The listing builds one solid part. Answer for the finished solid, in the listing's coordinates (mm). Coordinates: 2 decimals unless noted, no trailing zeros. Order: outer loops, then holes, each group sorted by start corner. A loop starts at its lowest first (then second) coordinate and runs counter-clockwise, first axis right, second up. Notation, with made-up numbers: (80, 31) - (92, 31) arc R13 cw to (92, 39) - close; hole circle Ø7 at (51.5, -33.75). An arc over 180 degrees is marked (long way). Use a Markdown table: item, result. Add a question column.
Item 1: Find the intervals of material crossed by line 1 along Y through (x, z) = (1.75, 8); line 2 along Y through (x, z) = (6.5, -23), in increasing order.
Item 2: Flat-ended cylindrical pins translate along their axes: P1, Ø3.5, axis at y = 23, z = 0, coming from the -X side; P2, Ø3, axis at x = 5.5, z = 13, coming from the +Y side; P3, Ø1, axis at x = 3, y = 30, coming from the -Z side. Find the tip coordinate at first contact, or state that the pin passes through.
Item 3: The part is cut by section A-A, the plane z = 0. Give the vertices of the cut face in (x, y).
Item 4: The part is cut by section B-B, the plane x = 6. State how many separate pieces and enclosed holes the cut face has, then the cut area to 3 significant figures.
from build123d import *

# Parameters (mm, degrees)
SPROCKET_R                   = 45.25
ESTRUSIONE_ESTRUSIONE2_DEPTH = 8
SCHIZZO1_R                   = 5
SCHIZZO1_R_2                 = 1.5
TAGLIO_ESTRUSIONE2_DEPTH     = 9
RACCORDO1_R                  = 0.5


with BuildPart() as part:
    # Sprocket → Estrusione-Estrusione2 (new body)
    with BuildSketch(Plane(origin=(0, 0, 0), x_dir=(0, 0, -1), z_dir=(1, 0, 0))):
        Circle(SPROCKET_R)
    extrude(amount=ESTRUSIONE_ESTRUSIONE2_DEPTH)

    # Schizzo1 → Taglio-Estrusione2 (cut, through all)
    with BuildSketch(Plane(origin=(0, 0, 0), x_dir=(0, 0, -1), z_dir=(1, 0, 0))):
        Circle(SCHIZZO1_R)
        with Locations((0, 23)):
            Circle(SCHIZZO1_R_2)
        with Locations((8, 0)):
            Circle(SCHIZZO1_R_2)
        with Locations((0, 8)):
            Circle(SCHIZZO1_R_2)
        with Locations((23, 0)):
            Circle(SCHIZZO1_R_2)
        with Locations((0, -8)):
            Circle(SCHIZZO1_R_2)
        with Locations((0, -23)):
            Circle(SCHIZZO1_R_2)
        with Locations((-8, 0)):
            Circle(SCHIZZO1_R_2)
        with Locations((-23, 0)):
            Circle(SCHIZZO1_R_2)
    extrude(amount=TAGLIO_ESTRUSIONE2_DEPTH, mode=Mode.SUBTRACT)

    # Raccordo1
    raccordo1_edges = [part.edges().sort_by_distance(p)[0] for p in [
        (0, 0, 45.25),
        (8, 0, 45.25),
    ]]
    fillet(raccordo1_edges, radius=RACCORDO1_R)


solid = part.part
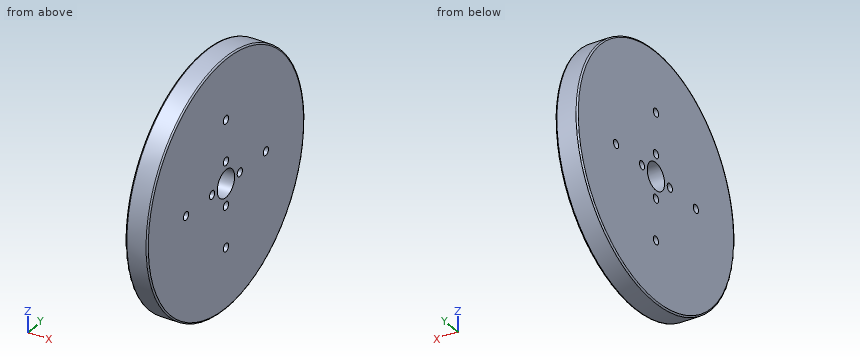
Solution:
| question | item | result |
|---|---|---|
| 1 | line 1 | y = -44.54 to -1.5, 1.5 to 44.54 |
| 1 | line 2 | y = -38.97 to -1.5, 1.5 to 38.97 |
| 2 | P1 | stops at x = 0 |
| 2 | P2 | stops at y = 43.76 |
| 2 | P3 | stops at z = -34.31 |
| 3 | outline | (0, -44.75) arc R0.5 ccw to (0.5, -45.25) - (7.5, -45.25) arc R0.5 ccw to (8, -44.75) - (8, -24.5) - (0, -24.5) - close; (0, -21.5) - (8, -21.5) - (8, -9.5) - (0, -9.5) - close; (0, -6.5) - (8, -6.5) - (8, -5) - (0, -5) - close; (0, 5) - (8, 5) - (8, 6.5) - (0, 6.5) - close; (0, 9.5) - (8, 9.5) - (8, 21.5) - (0, 21.5) - close; (0, 24.5) - (8, 24.5) - (8, 44.75) arc R0.5 ccw to (7.5, 45.25) - (0.5, 45.25) arc R0.5 ccw to (0, 44.75) - close |
| 4 | separate pieces | 1 |
| 4 | enclosed holes | 9 |
| 4 | area | 6,300 mm2 |
